```python
from build123d import *

# Parameters (mm, degrees)
SKETCH1_R                = 5.1
SKETCH1_R_2              = 1.75
BOSS_EXTRUDE1_DEPTH      = 3.5
SKETCH2_R                = 5.1
SKETCH2_R_2              = 4
BOSS_EXTRUDE2_DEPTH      = 1.5
BOSS_EXTRUDE2_DEPTH_BACK = 13.5


with BuildPart() as part:
    # Sketch1 → Boss-Extrude1 (new body)
    with BuildSketch(Plane.XY):
        with BuildLine():
            Line((-6.1, -9.153687781), (-6.1, 9.153687781))
            ThreePointArc((-6.1, 9.153687781), (0, 11), (6.1, 9.153687781))
            Line((6.1, 9.153687781), (6.1, -9.153687781))
            ThreePointArc((6.1, -9.153687781), (0, -11), (-6.1, -9.153687781))
        make_face()
        Circle(SKETCH1_R, mode=Mode.SUBTRACT)
        with Locations((0, 8)):
            Circle(SKETCH1_R_2, mode=Mode.SUBTRACT)
        with Locations((0, -8)):
            Circle(SKETCH1_R_2, mode=Mode.SUBTRACT)
    extrude(amount=-BOSS_EXTRUDE1_DEPTH)

    # Sketch2 → Boss-Extrude2 (add, two sides)
    with BuildSketch(Plane.XY) as boss_extrude2_sk:
        Circle(SKETCH2_R)
        Circle(SKETCH2_R_2, mode=Mode.SUBTRACT)
    extrude(amount=BOSS_EXTRUDE2_DEPTH)
    extrude(boss_extrude2_sk.sketch, amount=-BOSS_EXTRUDE2_DEPTH_BACK)


solid = part.part
```
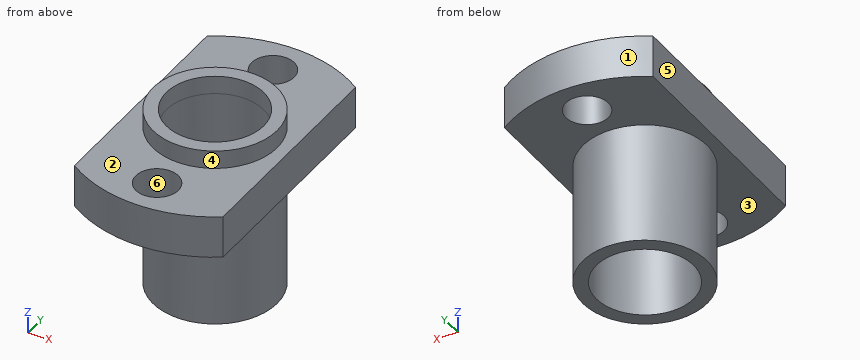
Can you work these out from the model? Positions are in its coordinate system, mm. Face numbers are marked on the shaded views. A direction names the side the tool comes from. Round coordinates to 2 decimals unless told otherwise and drop trailing zeros. Order: outer loops, then holes, each group sorted by start corner. A loop starts at its lowest first (then second) coordinate and runs counter-clockwise, first axis right, second up.
(1) If we section it at D-D (z = -10.25): Please give me the cut outline in (x, y), plus the area to 3 significant figures.
Results are:
outline: circle Ø10.2 at (0, 0); hole circle Ø8 at (0, 0)
area: 31.4 mm2
(2) If we section it at C-C (x = -3.75): Please give me the cut outline in (y, z), plus the area to 3 significant figures.
Results are:
outline: (-10.34, -3.5) - (-3.46, -3.5) - (-3.46, -13.5) - (-1.39, -13.5) - (-1.39, 1.5) - (-3.46, 1.5) - (-3.46, 0) - (-10.34, 0) - close; (1.39, -13.5) - (3.46, -13.5) - (3.46, -3.5) - (10.34, -3.5) - (10.34, 0) - (3.46, 0) - (3.46, 1.5) - (1.39, 1.5) - close
area: 110 mm2
(3) On a 3-axis mill with a long thin cutter (end or side, diameter ignored), from which of +Z, -Z, +X, -X, +Y, -Y can I reach the whole of each face in a straight line? I mean the marked faces 1, 2 and 3. Say none if no direction works.
Results are:
face 1: +Z, -Z, +Y
face 2: +Z
face 3: -Z
(4) We'd pull the mould along Y, two halves only. Please class the marked faces 4, 5 and 6: +Y half, -Y half, draft (parallel to the pull), parting line (faces both ways), or undercut.
Results are:
face 4: parting line
face 5: draft
face 6: undercut
(5) I'm going to push flat-ended pins straight in: pin 1 (5.5 mm diameter, centred on x = 0, y = 8, fed in from -Z); pin 2 (4.5 mm diameter, centred on x = 0, y = -8, fed in from +Z); pin 3 (3 mm diameter, centred on x = -0.5, y = -2.5, fed in from +Z); pin 4 (4 mm diameter, centred on x = 0, z = -11.5, fed in from -Y). Where does each tip first touch, or does it pass through?
Results are:
pin 1: stops at z = -3.5
pin 2: stops at z = 0
pin 3: stops at z = 1.5
pin 4: stops at y = -5.1
(6) If we section it at B-B (y = -8): Please give me the cut outline in (x, z).
Results are:
outline: (-6.1, -3.5) - (-1.75, -3.5) - (-1.75, 0) - (-6.1, 0) - close; (1.75, -3.5) - (6.1, -3.5) - (6.1, 0) - (1.75, 0) - close
(7) If we section it at A-A (x = 0): Please give me the cut outline in (y, z), plus the area to 3 significant figures.
Results are:
outline: (-11, -3.5) - (-9.75, -3.5) - (-9.75, 0) - (-11, 0) - close; (-6.25, -3.5) - (-5.1, -3.5) - (-5.1, -13.5) - (-4, -13.5) - (-4, 1.5) - (-5.1, 1.5) - (-5.1, 0) - (-6.25, 0) - close; (4, -13.5) - (5.1, -13.5) - (5.1, -3.5) - (6.25, -3.5) - (6.25, 0) - (5.1, 0) - (5.1, 1.5) - (4, 1.5) - close; (9.75, -3.5) - (11, -3.5) - (11, 0) - (9.75, 0) - close
area: 49.8 mm2
(8) If I drill on L1, parallel to Y at x = 0, z = -5; L2, parallel to Z at x = 4.25, y = 8.5; L3, parallel to X at y = 2, z = -5.5, over which ranges is the centre line in solid material (lowest first)?
Results are:
L1: y = -5.1 to -4, 4 to 5.1
L2: z = -3.5 to 0
L3: x = -4.69 to -3.46, 3.46 to 4.69
